Part model, mm, in its own coordinate system. A direction names the side the tool comes from. Give positions to 0.01 mm unless a question says otherwise; leave off trailing zeros. Write each loop counter-clockwise with the first axis right and the second up, starting at its lowest first coordinate (ties: lowest second). Pieces come first, ordered by that corner, then holes. Notation, with made-up numbers: (-1, 7.25) - (25, 7.25) arc R14 ccw to (25, 11.25) - close; hole circle Ø9 at (17, -15.5). An arc over 180 degrees is marked (long way). Answer in a Markdown table with one row per item. Add a question column.
1. Which spindle directions (+Z, -Z, +X, -X, +Y, -Y) get a long thin tool onto all of the face, cutting with end or side? Do faces 5 (the flat face through (0, -68, 32)), 6 (the flat face through (2, 36, 20)), 7 (the flat face through (2, 105, 6)). Say none if no direction does.
2. Band-saw the part on C-C on x = 2.2. Write the cut outline in (y, z).
3. Band-saw the part on B-B on y = 105.5. Write the cut outline in (x, z).
4. Pull direction Y, two halves, no side cores. Call faces 1 (the flat face through (2, 105, 14)), 2 (the flat face through (2, -107.5, 70)), 3 (the flat face through (5, -68, 32)), 4 (the cylindrical face through (2, 128, 1)): released by +Y, released by -Y, zero draft, split by the parting line, or undercut.
5. Band-saw the part on D-D on z = 78. Write the cut outline in (x, y), plus the area to 3 significant figures.
6. Probe line 1 along Y through (x, z) = (0.9, 75); line 2 along Z through (x, y) = (3.75, 91); line 3 along Y through (x, z) = (4.35, 51). List the from-to ranges inside material, lowest first.
7. Band-saw the part on A-A on z = 10. Write the cut outline in (x, y), plus the area to 3 significant figures.
8. Drop flat-ended pins along their axis: pin 1 Ø1.5 at (x, z) = (2, 70) entering from +Y; pin 2 Ø1.5 at (x, y) = (2.5, 108) entering from +Z. Give the stop position or say it passes through.
```python
from build123d import *

# Parameters (mm, degrees)
F1_DEPTH = 5


with BuildPart() as f1:
    # F0 (on Right) → F1 (new body)
    with BuildSketch(Plane.YZ):
        with BuildLine():
            ThreePointArc((-125, 100), (-128.535534, 98.535534), (-130, 95))
            Line((-130, 95), (-130, 5))
            ThreePointArc((-130, 5), (-128.535534, 1.464466), (-125, 0))
            Line((-125, 0), (125, 0))
            ThreePointArc((125, 0), (128.535534, 1.464466), (130, 5))
            Line((130, 5), (130, 15))
            ThreePointArc((130, 15), (128.535534, 18.535534), (125, 20))
            Line((125, 20), (-55, 20))
            ThreePointArc((-55, 20), (-58.535534, 21.464466), (-60, 25))
            Line((-60, 25), (-60, 95))
            ThreePointArc((-60, 95), (-61.464466, 98.535534), (-65, 100))
            Line((-65, 100), (-125, 100))
        make_face()
        with BuildLine():
            Line((90, 14), (120, 14))
            ThreePointArc((120, 14), (124, 10), (120, 6))
            Line((120, 6), (90, 6))
            ThreePointArc((90, 6), (86, 10), (90, 14))
        make_face(mode=Mode.SUBTRACT)
        with BuildLine():
            ThreePointArc((-117.5, 85), (-112.5, 90), (-107.5, 85))
            Line((-107.5, 85), (-107.5, 55))
            ThreePointArc((-107.5, 55), (-112.5, 50), (-117.5, 55))
            Line((-117.5, 55), (-117.5, 85))
        make_face(mode=Mode.SUBTRACT)
        with BuildLine():
            ThreePointArc((-82.5, 85), (-77.5, 90), (-72.5, 85))
            Line((-72.5, 85), (-72.5, 55))
            ThreePointArc((-72.5, 55), (-77.5, 50), (-82.5, 55))
            Line((-82.5, 55), (-82.5, 85))
        make_face(mode=Mode.SUBTRACT)
    extrude(amount=F1_DEPTH)


solid = f1.part
```
Values:
| question | item | result |
|---|---|---|
| 1 | face 5 | +Z, -Z, -X, +Y, -Y |
| 1 | face 6 | +Z, +X, -X, +Y |
| 1 | face 7 | +X, -X |
| 2 | outline | (-130, 5) arc R5 ccw to (-125, 0) - (125, 0) arc R5 ccw to (130, 5) - (130, 15) arc R5 ccw to (125, 20) - (-55, 20) arc R5 cw to (-60, 25) - (-60, 95) arc R5 ccw to (-65, 100) - (-125, 100) arc R5 ccw to (-130, 95) - close; hole (-117.5, 55) arc R5 ccw to (-107.5, 55) - (-107.5, 85) arc R5 ccw to (-117.5, 85) - close; hole (-82.5, 55) arc R5 ccw to (-72.5, 55) - (-72.5, 85) arc R5 ccw to (-82.5, 85) - close; hole (90, 6) - (120, 6) arc R4 ccw to (120, 14) - (90, 14) arc R4 ccw to start |
| 3 | outline | (0, 0) - (5, 0) - (5, 6) - (0, 6) - close; (0, 14) - (5, 14) - (5, 20) - (0, 20) - close |
| 4 | face 1 | undercut |
| 4 | face 2 | undercut |
| 4 | face 3 | zero draft |
| 4 | face 4 | released by +Y |
| 5 | outline | (0, -130) - (5, -130) - (5, -117.5) - (0, -117.5) - close; (0, -107.5) - (5, -107.5) - (5, -82.5) - (0, -82.5) - close; (0, -72.5) - (5, -72.5) - (5, -60) - (0, -60) - close |
| 5 | area | 250 mm² |
| 6 | line 1 | y = -130 to -117.5, -107.5 to -82.5, -72.5 to -60 |
| 6 | line 2 | z = 0 to 6, 14 to 20 |
| 6 | line 3 | y = -130 to -115.5, -109.5 to -80.5, -74.5 to -60 |
| 7 | outline | (0, -130) - (5, -130) - (5, 86) - (0, 86) - close; (0, 124) - (5, 124) - (5, 130) - (0, 130) - close |
| 7 | area | 1,110 mm² |
| 8 | pin 1 | stops at y = -60 |
| 8 | pin 2 | stops at z = 20 |
